Read the model definition and answer for the solid it produces. Units are mm, in the model's axes. Face numbers are marked on the shaded views. A direction names the side the tool comes from. Coordinates: 2 decimals unless noted, no trailing zeros. Order: outer loops, then holes, each group sorted by start corner. A loop starts at its lowest first (then second) coordinate and runs counter-clockwise, first axis right, second up. Notation, with made-up numbers: (-32.5, 11.25) -> (12.5, 11.25) arc R19 cw to (12.5, 48.25) -> close; hole circle Ø3 at (-13.75, 11). An arc over 180 degrees is marked (long way). Answer as a JSON object with one key per item and string values. Group by question number.
1) Section C-C on z = 14 is taken. Determine the outline of the cut face in (x, y), and give its area (3 significant figures).
2) Consider L1, parallel to Z at x = -31.75, y = 0; L2, parallel to Z at x = -31, y = 16.5; L3, parallel to X at y = 7.5, z = 8. Determine where each line is inside the solid, lowest interval first.
3) Section D-D on x = 0 is taken. Determine the outline of the cut face in (y, z).
4) Section A-A on y = 0 is taken. Determine the outline of the cut face in (x, z).
5) Given pin 1 (12 mm diameter, centred on x = 35.5, y = -18, fed in from +Z); pin 2 (16 mm diameter, centred on y = 3, z = 45.5, fed in from -X); pin 3 (1.5 mm diameter, centred on y = -3.5, z = 29.5, fed in from +X), each flat-ended and moving along its own axis, determine where each tip first touches the part or whether it passes through.
6) A tool of negligible diameter and unlimited length cuts with its end or side. For the marked faces 1, 2, 3 and 4, from which of +Z, -Z, +X, -X, +Y, -Y can it reach the whole face along a straight path? Write none if from no direction.
7) Section B-B on z = 42 is taken. Determine the outline of the cut face in (x, y), and give its area (3 significant figures).
8) Determine the mould class of the marked faces 5, 6, 7 and 8 for opening direction Z: released by +Z, released by -Z, zero draft, split by the parting line, or undercut.
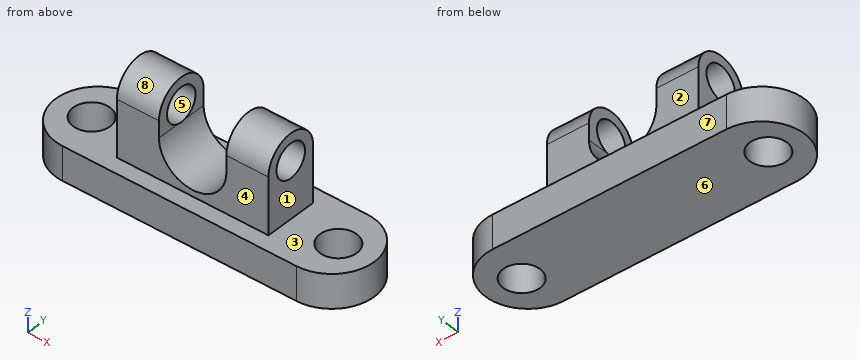
from build123d import *

# Parameters (mm, degrees)
F1_DEPTH  = 20.32
F2_R      = 11.1083186408
F3_DEPTH  = 25.4
F4_W      = 91.2809744477
F4_H      = 32.0040024817
F5_DEPTH  = 34.036
F6_R      = 16.0020012408
F7_DEPTH  = 91.2809744477
F9_DEPTH  = 33.528
F10_R     = 10.2254227484
F11_DEPTH = 105.41


with BuildPart() as f1:
    # F0 (on Top) → F1 (new body)
    with BuildSketch(Plane.XY):
        with BuildLine():
            ThreePointArc((70.4088062048, -25.4640523344), (95.8728585392, 0), (70.4088062048, 25.4640523344))
            Line((70.4088062048, 25.4640523344), (-70.4088062048, 25.4640523344))
            ThreePointArc((-70.4088062048, 25.4640523344), (-95.8728585392, 0), (-70.4088062048, -25.4640523344))
            Line((-70.4088062048, -25.4640523344), (70.4088062048, -25.4640523344))
        make_face()
    extrude(amount=F1_DEPTH)

    # F2 (on face) → F3 (cut)
    with BuildSketch(Plane.XY.offset(20.32)):
        with Locations((74.3049383163, 0)):
            Circle(F2_R)
        with Locations((-74.3049383163, 0)):
            Circle(F2_R)
    extrude(amount=-F3_DEPTH, mode=Mode.SUBTRACT)

    # F4 (on face) → F5 (join)
    with BuildSketch(Plane.XY.offset(20.32)):
        Rectangle(F4_W, F4_H)
    extrude(amount=F5_DEPTH)

    # F6 (on face) → F7 (join, through all)
    with BuildSketch(Plane.YZ.offset(45.6404872239)):
        with Locations((0, 54.356)):
            Circle(F6_R)
    extrude(amount=-F7_DEPTH)

    # F8 (on Front) → F9 (cut, symmetric)
    with BuildSketch(Plane.XZ):
        with BuildLine():
            Line((20.3155819327, 44.3881601095), (20.3155819327, 96.7077314854))
            Line((20.3155819327, 96.7077314854), (-20.3155819327, 96.7077314854))
            Line((-20.3155819327, 96.7077314854), (-20.3155819327, 44.3881601095))
            ThreePointArc((-20.3155819327, 44.3881601095), (0, 24.0725781769), (20.3155819327, 44.3881601095))
        make_face()
    extrude(amount=F9_DEPTH, both=True, mode=Mode.SUBTRACT)

    # F10 (on face) → F11 (cut)
    with BuildSketch(Plane.YZ.offset(45.6404872239)):
        with Locations((0, 54.356)):
            Circle(F10_R)
    extrude(amount=-F11_DEPTH, mode=Mode.SUBTRACT)


solid = f1.part
Worked answers:
{
 "1": {"outline": "(-70.41, -25.46) -> (70.41, -25.46) arc R25.46 ccw to (70.41, 25.46) -> (-70.41, 25.46) arc R25.46 ccw to start; hole circle Ø22.22 at (-74.3, 0); hole circle Ø22.22 at (74.3, 0)", "area": "8,430 mm²"},
 "2": {"L1": "z = 0 to 44.13, 64.58 to 70.36", "L2": "z = 0 to 20.32", "L3": "x = -94.74 to -82.5, -66.11 to 66.11, 82.5 to 94.74"},
 "3": {"outline": "(-25.46, 0) -> (25.46, 0) -> (25.46, 20.32) -> (16, 20.32) -> (16, 24.07) -> (-16, 24.07) -> (-16, 20.32) -> (-25.46, 20.32) -> close"},
 "4": {"outline": "(-95.87, 0) -> (-85.41, 0) -> (-85.41, 20.32) -> (-95.87, 20.32) -> close; (-63.2, 0) -> (63.2, 0) -> (63.2, 20.32) -> (45.64, 20.32) -> (45.64, 44.13) -> (20.31, 44.13) arc R20.32 cw to (-20.31, 44.13) -> (-45.64, 44.13) -> (-45.64, 20.32) -> (-63.2, 20.32) -> close; (-45.64, 64.58) -> (-20.32, 64.58) -> (-20.32, 70.36) -> (-45.64, 70.36) -> close; (20.32, 64.58) -> (45.64, 64.58) -> (45.64, 70.36) -> (20.32, 70.36) -> close; (85.41, 0) -> (95.87, 0) -> (95.87, 20.32) -> (85.41, 20.32) -> close"},
 "5": {"pin 1": "stops at z = 64.94", "pin 2": "stops at x = -45.64", "pin 3": "stops at x = 45.64"},
 "6": {"face 1": "+Z, +X, +Y, -Y", "face 2": "+Z, +X, -X, +Y", "face 3": "+Z", "face 4": "+Z, +X, -X, -Y"},
 "7": {"outline": "(-45.64, -16) -> (-20.17, -16) -> (-20.17, 16) -> (-45.64, 16) -> close; (20.17, -16) -> (45.64, -16) -> (45.64, 16) -> (20.17, 16) -> close", "area": "1,630 mm²"},
 "8": {"face 5": "undercut", "face 6": "released by -Z", "face 7": "zero draft", "face 8": "released by +Z"}
}
